Part print with two shaded views. Sizes in mm from the minimum x, y, z corner. A direction names the side the tool comes from. Coordinates: 2 decimals unless noted, no trailing zeros. Loops run counter-clockwise (first coordinate to the right, second up) from the corner with the lowest first, then second, coordinate; pieces in that order, holes last. Notation, with made-up numbers: (85, 1) -> (142, 1) arc R34 cw to (142, 32) -> close; hole circle Ø4 at (39, 75). An arc over 180 degrees is marked (long way). Return JSON: item names as keys, results as strings. Group by question number.
(1) Tool access for the marked faces 1 and 2: list every direction of +Z, -Z, +X, -X, +Y, -Y with a clear straight run to the whole face (end or side of a thin tool).
(2) Saw through at B-B on z = 14. Write the cut outline in (x, y).
(3) Flat gauge pins, fed straight in: pin 1 Ø4 at (y, z) = (25, 32.5) entering from +X; pin 2 Ø5 at (y, z) = (39.5, 31) entering from -X; pin 3 Ø10 at (y, z) = (37, 34) entering from -X. Where does each tip first touch, or does it go through?
(4) Saw through at D-D on z = 38. Write the cut outline in (x, y), then the cut area to 3 significant figures.
(5) Saw through at A-A on x = 30. Write the cut outline in (y, z).
(6) Mould opens along X. For the marked faces 3, 4 and 5 say: pulls with the +X half, pulls with the -X half, needs draft (parallel to the pull), parting line crosses it, or undercut.
(7) Probe L1, parallel to Y at x = 30, z = 26; L2, parallel to Y at x = 42, z = 6; L3, parallel to X at y = 33, z = 31. List the from-to ranges inside material, lowest first.
(8) Saw through at C-C on y = 27.5. Give the number of separate pieces and of enclosed holes in the cut face, then the cut area to 3 significant figures.
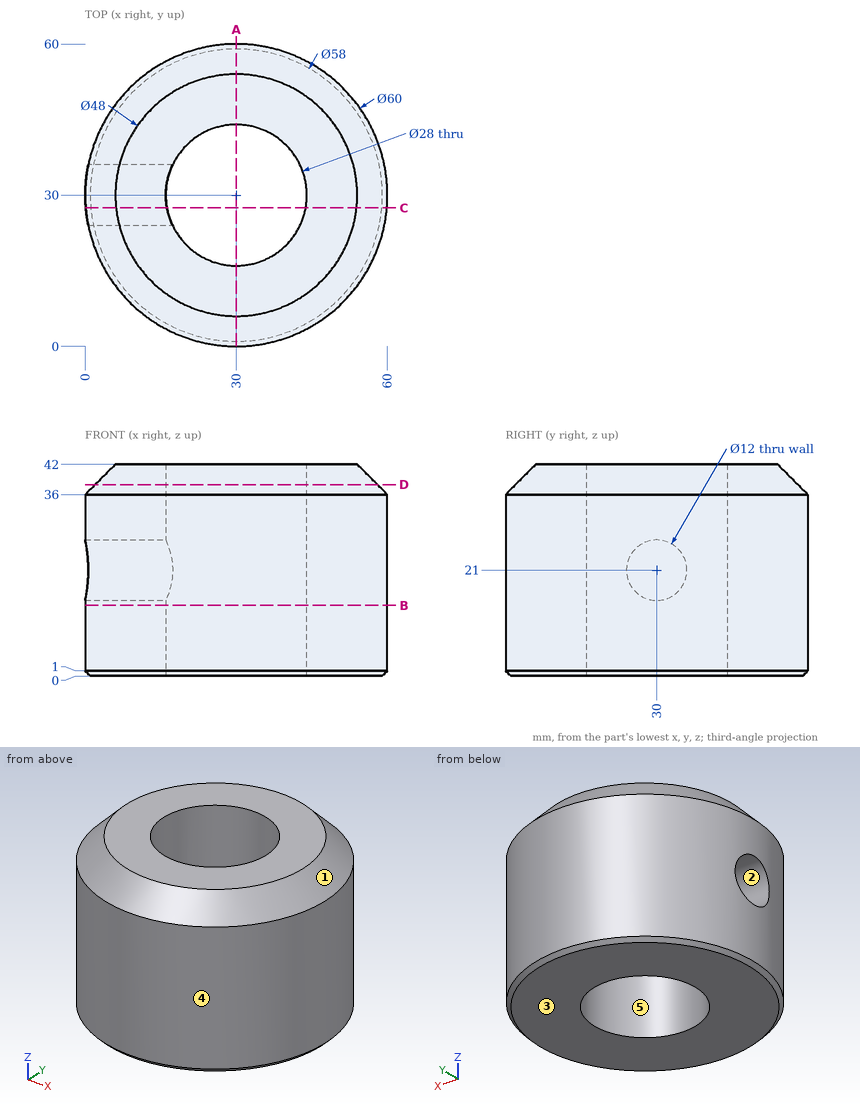
Geometry results:
{
 "1": {"face 1": "+Z", "face 2": "-X"},
 "2": {"outline": "circle Ø60 at (30, 30); hole circle Ø28 at (30, 30)"},
 "3": {"pin 1": "x = 59.85", "pin 2": "x = 0.83", "pin 3": "x = 0.07"},
 "4": {"outline": "circle Ø56 at (30, 30); hole circle Ø28 at (30, 30)", "area": "1,850 mm²"},
 "5": {"outline": "(0, 1) -> (1, 0) -> (16, 0) -> (16, 42) -> (6, 42) -> (0, 36) -> close; (44, 0) -> (59, 0) -> (60, 1) -> (60, 36) -> (54, 42) -> (44, 42) -> close"},
 "6": {"face 3": "needs draft", "face 4": "parting line crosses it", "face 5": "undercut"},
 "7": {"L1": "0 to 16, 44 to 60", "L2": "2.5 to 22.79, 37.21 to 57.5", "L3": "0.15 to 16.33, 43.67 to 59.85"},
 "8": {"separate pieces": "3", "enclosed holes": "0", "area": "1,140 mm²"}
}
